CAD build for the part. Positions are in the model's coordinates, mm. Face numbers are marked on the shaded views. Give positions to 0.01 mm unless a question says otherwise; leave off trailing zeros. Write each loop counter-clockwise with the first axis right and the second up, starting at its lowest first coordinate (ties: lowest second). Pieces come first, ordered by that corner, then holes. Notation, with made-up numbers: (75, -25.5) - (109, -25.5) arc R19 ccw to (109, 7.5) - close; hole circle Ø10 at (35.5, -17). An arc over 180 degrees is marked (long way). Put each result on its own line as item: value. Start each with the question number.
1. Drop flat-ended pins along their axis: pin 1 (10 mm diameter, centred on x = -0.5, z = 13.5, fed in from -Y); pin 2 (1 mm diameter, centred on y = -1.5, z = 9, fed in from +X); pin 3 (11 mm diameter, centred on x = 11.5, z = 12, fed in from -Y). Give the stop position or say it passes through.
2. Cut at D-D on z = 2.5. List the corners of the cut face in (x, y), and give its area (3 significant figures).
3. Mould opens along Y. For the marked faces 1, 2 and 3 say: +Y half, -Y half, draft (parallel to the pull), parting line (faces both ways), or undercut.
4. Cut at B-B on x = 3. List the corners of the cut face in (y, z).
5. Cut at C-C on z = 23.5. List the corners of the cut face in (x, y).
6. Cut at A-A on y = 0. List the corners of the cut face in (x, z), and give its area (3 significant figures).
7. Wall check: line 1 (Z direction, x = 11, y = 4.85); line 2 (Y direction, x = 5.5, z = 11.75); line 3 (X direction, y = 0, z = 10). Give the ranges that are in metal, low to high.
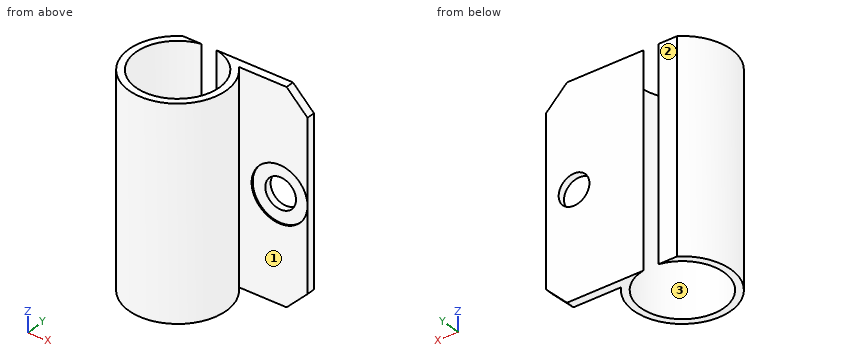
from build123d import *

# Parameters (mm, degrees)
SKETCH_R        = 7
SKETCH_R_2      = 6
PAD_DEPTH       = 30
SKETCH001_W     = 21.169265
SKETCH001_H     = 5.002638
POCKET_DEPTH    = 30.001
SKETCH002_W     = 11.233038
SKETCH002_H     = 30
SKETCH002_R     = 2.2
PAD001_DEPTH    = 1.2
SKETCH003_R     = 4
POCKET001_DEPTH = 0.2
CHAMFER_SIZE    = 3


with BuildPart() as part:
    # Sketch → Pad (new body)
    with BuildSketch(Plane.XY):
        Circle(SKETCH_R)
        Circle(SKETCH_R_2, mode=Mode.SUBTRACT)
    extrude(amount=PAD_DEPTH)

    # Sketch001 → Pocket (cut, through all)
    with BuildSketch(Plane.XY.offset(30)):
        with Locations((-0.201503, 8.401319)):
            Rectangle(SKETCH001_W, SKETCH001_H)
    extrude(amount=-POCKET_DEPTH, mode=Mode.SUBTRACT)

    # Sketch002 → Pad001 (new body)
    with BuildSketch(Plane(origin=(0, 5.9, 0), x_dir=(-1, 0, 0), z_dir=(0, 1, 0))):
        with Locations((-9.383481, 15)):
            Rectangle(SKETCH002_W, SKETCH002_H)
        with Locations((-11, 15)):
            Circle(SKETCH002_R, mode=Mode.SUBTRACT)
    extrude(amount=-PAD001_DEPTH)

    # Sketch003 → Pocket001 (cut)
    with BuildSketch(Plane.XZ.offset(-4.7)):
        with Locations((11, 15)):
            Circle(SKETCH003_R)
    extrude(amount=-POCKET001_DEPTH, mode=Mode.SUBTRACT)

    # Chamfer
    chamfer_edges = [part.edges().sort_by_distance(p)[0] for p in [
        (15, 5.3, 0),
        (15, 5.3, 30),
    ]]
    chamfer(chamfer_edges, length=CHAMFER_SIZE)


solid = part.part
Report:
1. pin 1: stops at y = -7
1. pin 2: stops at x = 6.93
1. pin 3: stops at y = -3.61
2. outline: (-3.77, 5.9) arc R7 ccw (long way) to (5.19, 4.7) - (14.5, 4.7) - (14.5, 5.9) - (1.09, 5.9) arc R6 cw (long way) to (-1.09, 5.9) - close
2. area: 47.3 mm²
3. face 1: undercut
3. face 2: +Y half
3. face 3: undercut
4. outline: (-6.32, 0) - (-5.2, 0) - (-5.2, 30) - (-6.32, 30) - close; (5.2, 0) - (5.9, 0) - (5.9, 30) - (5.2, 30) - close
5. outline: (-3.77, 5.9) arc R7 ccw (long way) to (5.19, 4.7) - (15, 4.7) - (15, 5.9) - (1.09, 5.9) arc R6 cw (long way) to (-1.09, 5.9) - close
6. outline: (-7, 0) - (-6, 0) - (-6, 30) - (-7, 30) - close; (6, 0) - (7, 0) - (7, 30) - (6, 30) - close
6. area: 60.0 mm²
7. line 1: z = 0 to 11, 19 to 30
7. line 2: y = -4.33 to -2.4, 2.4 to 4.33, 4.7 to 5.9
7. line 3: x = -7 to -6, 6 to 7
